```python
from build123d import *

# Parameters (mm, degrees)
SKETCH1_W                     = 150
SKETCH1_H                     = 65
BOSS_EXTRUDE1_DEPTH           = 20
SKETCH4_W                     = 130
SKETCH4_H                     = 45
CUT_EXTRUDE1_DEPTH            = 10
M2_5_TAPPED_HOLE1_D           = 2.05
M2_5_TAPPED_HOLE1_DEPTH       = 8
M2_5_TAPPED_HOLE1_CSINK_D     = 2.55
M2_5_TAPPED_HOLE1_CSINK_ANGLE = 90
M2_5_TAPPED_HOLE1_TIP         = 0.615882135
FILLET1_R                     = 2
FILLET2_R                     = 2
M2_5_TAPPED_HOLE2_D           = 2.05
M2_5_TAPPED_HOLE2_DEPTH       = 8
M2_5_TAPPED_HOLE2_CSINK_D     = 2.55
M2_5_TAPPED_HOLE2_CSINK_ANGLE = 90
M2_5_TAPPED_HOLE2_TIP         = 0.615882135
CHAMFER1_SIZE                 = 1


with BuildPart() as part:
    # Sketch1 → Boss-Extrude1 (new body)
    with BuildSketch(Plane(origin=(0, 0, 0), x_dir=(1, 0, 0), z_dir=(0, 1, 0))):
        Rectangle(SKETCH1_W, SKETCH1_H)
    extrude(amount=BOSS_EXTRUDE1_DEPTH)

    # Sketch3 → 1/8 NPT Tapped Hole1 (revolve, cut)
    with BuildSketch(Plane(origin=(60, 0, 0), x_dir=(0, 0, -1), z_dir=(1, 0, 0))):
        Polygon((0, 0), (0, 20), (4.2164, 20), (4.2164, 6.92), (4.537398933, 6.92), (4.744593, 0), align=None)
    revolve(axis=Axis((60, -6.35, 0), (0, 1, 0)), mode=Mode.SUBTRACT)

    # Sketch4 → Cut-Extrude1 (cut)
    with BuildSketch(Plane(origin=(0, 20, 0), x_dir=(1, 0, 0), z_dir=(0, 1, 0))):
        Rectangle(SKETCH4_W, SKETCH4_H)
    extrude(amount=-CUT_EXTRUDE1_DEPTH, mode=Mode.SUBTRACT)

    # M2.5 Tapped Hole1
    with Locations(Plane(origin=(-70, 20, -17.5), x_dir=(0, 0, 1), z_dir=(0, 1, 0))):
        with Locations((0, 0), (11.666666667, 0), (23.333333333, 0), (35, 0), (45, 10), (45, 27.142857143), (45, 44.285714286), (45, 61.428571429), (45, 78.571428571), (45, 95.714285714), (45, 112.857142857), (45, 130), (-10, 10), (-10, 27.142857143), (-10, 44.285714286), (-10, 61.428571429), (-10, 78.571428571), (-10, 95.714285714), (-10, 112.857142857), (-10, 130), (0, 140), (11.666666667, 140), (23.333333333, 140), (35, 140), (-10, 140), (45, 140), (-10, 0), (45, 0)):
            CounterSinkHole(M2_5_TAPPED_HOLE1_D / 2, M2_5_TAPPED_HOLE1_CSINK_D / 2, depth=M2_5_TAPPED_HOLE1_DEPTH, counter_sink_angle=M2_5_TAPPED_HOLE1_CSINK_ANGLE)
            with Locations((0, 0, -(M2_5_TAPPED_HOLE1_DEPTH + M2_5_TAPPED_HOLE1_TIP / 2))):  # 118° drill point
                Cone(0, M2_5_TAPPED_HOLE1_D / 2, M2_5_TAPPED_HOLE1_TIP, mode=Mode.SUBTRACT)

    # Fillet1
    fillet1_edges = [part.edges().sort_by_distance(p)[0] for p in [
        (-75, 10, -32.5),
        (75, 10, -32.5),
        (75, 10, 32.5),
        (-75, 10, 32.5),
    ]]
    fillet(fillet1_edges, radius=FILLET1_R)

    # Fillet2
    fillet2_edges = [part.edges().sort_by_distance(p)[0] for p in [
        (-65, 15, -22.5),
        (65, 15, -22.5),
        (65, 15, 22.5),
        (-65, 15, 22.5),
    ]]
    fillet(fillet2_edges, radius=FILLET2_R)

    # M2.5 Tapped Hole2
    with Locations(Plane(origin=(-42.75, 0, 7), x_dir=(0, 0, -1), z_dir=(0, -1, 0))):
        with Locations((0, 0), (0, 55.5), (14, 0), (14, 55.5)):
            CounterSinkHole(M2_5_TAPPED_HOLE2_D / 2, M2_5_TAPPED_HOLE2_CSINK_D / 2, depth=M2_5_TAPPED_HOLE2_DEPTH, counter_sink_angle=M2_5_TAPPED_HOLE2_CSINK_ANGLE)
            with Locations((0, 0, -(M2_5_TAPPED_HOLE2_DEPTH + M2_5_TAPPED_HOLE2_TIP / 2))):  # 118° drill point
                Cone(0, M2_5_TAPPED_HOLE2_D / 2, M2_5_TAPPED_HOLE2_TIP, mode=Mode.SUBTRACT)

    # Chamfer1
    chamfer1_edges = [part.edges().sort_by_distance(p)[0] for p in [
        (0, 0, -32.5),
        (-75, 0, 0),
        (75, 0, 0),
        (0, 0, 32.5),
        (-74.414213562, 0, -31.914213562),
        (-74.414213562, 0, 31.914213562),
        (74.414213562, 0, 31.914213562),
        (74.414213562, 0, -31.914213562),
    ]]
    chamfer(chamfer1_edges, length=CHAMFER1_SIZE)


solid = part.part
```
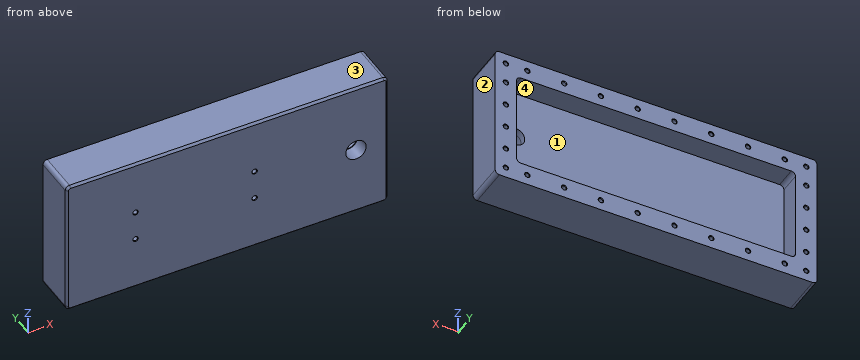
Work out the finished part from the listing and answer in its coordinate system (mm). Face numbers are marked on the shaded views. Give positions to 0.01 mm unless a question says otherwise; leave off trailing zeros. Write each loop counter-clockwise with the first axis right and the second up, starting at its lowest first coordinate (ties: lowest second). Pieces come first, ordered by that corner, then holes.
(1) The part is cut by section B-B on x = 47.5. Write down the section's boundary in (y, z).
Final values:
outline: (0, -31.5) - (1, -32.5) - (20, -32.5) - (20, -22.5) - (10, -22.5) - (10, 22.5) - (20, 22.5) - (20, 32.5) - (1, 32.5) - (0, 31.5) - close
(2) The part is cut by section A-A on z = 0. Write down the section's boundary in (x, y), plus the area to 3 significant figures.
Final values:
outline: (-75, 1) - (-74, 0) - (55.26, 0) - (55.46, 6.92) - (55.78, 6.92) - (55.78, 10) - (-65, 10) - (-65, 20) - (-75, 20) - close; (64.22, 6.92) - (64.54, 6.92) - (64.74, 0) - (74, 0) - (75, 1) - (75, 20) - (65, 20) - (65, 10) - (64.22, 10) - close
area: 1,610 mm2
(3) The part is cut by section C-C on y = 17. Count the separate pieces of the cut face and the enclosed holes in it, plus the area to 3 significant figures.
Final values:
separate pieces: 1
enclosed holes: 29
area: 3,810 mm2
(4) The mould has two halves that part along X. Classify the marked faces 1, 2, 3 and 4: pulls with the +X half, pulls with the -X half, needs draft (parallel to the pull), parting line crosses it, or undercut.
Final values:
face 1: undercut
face 2: pulls with the +X half
face 3: needs draft
face 4: undercut
(5) Flat-ended cylindrical pins translate along their axes: pin 1 Ø6 at (x, z) = (3.5, -10.5) entering from +Y; pin 2 Ø1.2 at (x, z) = (-8.57, 27.5) entering from +Y; pin 3 Ø1.2 at (x, z) = (70, -17.5) entering from -Y; pin 4 Ø1.6 at (x, z) = (-70, -17.5) entering from +Y. Find the tip coordinate at first contact, or state that the pin passes through.
Final values:
pin 1: stops at y = 10
pin 2: stops at y = 11.75
pin 3: stops at y = 0
pin 4: stops at y = 11.86
(6) Straight lines are drawn through the part: line 1 (X direction, y = 4.5, z = 7) (3 decimals); line 2 (Z direction, x = -60, y = 17.75) (3 decimals); line 3 (Z direction, x = 13, y = 5.5). For each, find the intervals that lie inside material, in ascending order.
Final values:
line 1: x = -75 to -43.775, -41.725 to 11.725, 13.775 to 75
line 2: z = -32.5 to -28.525, -26.475 to -22.5, 22.5 to 26.475, 28.525 to 32.5
line 3: z = -32.5 to -7.99, -6.01 to 6.01, 7.99 to 32.5
